```python
from build123d import *

# Parameters (mm, degrees)
SKETCH002_R  = 2.25
POCKET_DEPTH = 31.001
CHAMFER_SIZE = 2.5


with BuildPart() as chamfer_body:
    # Sketch → Loft section 0
    with BuildSketch(Plane.XY):
        with BuildLine():
            Line((-17, 0), (-38, 0))
            Line((-38, 0), (-38, -6))
            Line((-38, -6), (-20, -6))
            ThreePointArc((-16.27755, -9.477078), (-17.453105, -7.004482), (-20, -6))
            Line((-16.27755, -9.477078), (-15, -28.197751))
            ThreePointArc((-15, -28.197751), (-14.052596, -30.190467), (-12, -31))
            Line((-12, -31), (0, -31))
            Line((0, -31), (0, -27))
            ThreePointArc((-9.789322, -18.64486), (-6.435045, -24.627224), (0, -27))
            Line((-11.683183, -4.645958), (-9.789322, -18.64486))
            ThreePointArc((-11.683183, -4.645958), (-13.469651, -1.325133), (-17, 0))
        make_face()
    # Sketch001 → Loft section 1
    with BuildSketch(Plane.XY.offset(20)):
        with BuildLine():
            Line((-17, 0), (-38, 0))
            Line((-38, 0), (-38, -6))
            Line((-38, -6), (-16.5, -6))
            ThreePointArc((-12.77755, -9.220661), (-14.038837, -6.91692), (-16.5, -6))
            Line((-12.77755, -9.220661), (-11.623745, -17.1614))
            ThreePointArc((-11.623745, -17.1614), (-9.823458, -22.15833), (-6, -25.844998))
            ThreePointArc((-6, -25.844998), (-3.112034, -27.078665), (0, -27.5))
            Line((0, -27.5), (0, -24.5))
            ThreePointArc((-8.696641, -16.14486), (-6.029924, -22.072766), (0, -24.5))
            Line((-10.286118, -5.764115), (-8.696641, -16.14486))
            ThreePointArc((-10.286118, -5.764115), (-12.575601, -1.638712), (-17, 0))
        make_face()
    loft()

    # Sketch002 → Pocket (cut, through all)
    with BuildSketch(Plane(origin=(0, 0, 0), x_dir=(-1, 0, 0), z_dir=(0, 1, 0))):
        with Locations((23, 13.5)):
            Circle(SKETCH002_R)
        with Locations((31, 6.5)):
            Circle(SKETCH002_R)
    extrude(amount=-POCKET_DEPTH, mode=Mode.SUBTRACT)

    # Chamfer
    chamfer_edges = [chamfer_body.edges().sort_by_distance(p)[0] for p in [
        (-21.369261, -6, 15.050223),
        (-24.630739, -6, 11.949777),
        (-28.776606, -6, 6.844988),
        (-33.223394, -6, 6.155012),
    ]]
    chamfer(chamfer_edges, length=CHAMFER_SIZE)


with BuildPart() as part_mirroring:
    # Part__Mirroring: instance of Chamfer body
    add(chamfer_body.part.mirror(Plane(origin=(0, 0, 0), x_dir=(0, -1, 0), z_dir=(1, 0, 0))))


with BuildPart() as fusion:
    # Fusion base: copy of Chamfer body
    add(chamfer_body.part)

    # Fusion: union Part__Mirroring
    add(part_mirroring.part)


solid = fusion.part
```
Here's how the part is built. I have some questions about the finished solid (model axes, mm). Coordinates: 2 decimals unless noted, no trailing zeros. Return JSON: item names as keys, results as strings.
1) If we section it at A-A, the plane z = 12.25: Count the separate pieces of the cut face and the enclosed holes in it, then the cut area to 3 significant figures.
Results below:
{"separate pieces": "3", "enclosed holes": "0", "area": "500 mm²"}
2) Thinking about a two-plate mould opening in Z: for faces 1 (the face through (-27, 0, 10)), 2 (the face through (-25.146, -1.726, 14.176)), 3 (the face through (11, -9, 20)), which applies, +Z half, -Z half, draft (parallel to the pull), parting line (faces both ways), or undercut?
Results below:
{"face 1": "draft", "face 2": "undercut", "face 3": "+Z half"}
3) Will these pins go through, and if not, where does the flat tip stop? pin 1 (3 mm diameter, centred on y = -25, z = 11, fed in from -X); pin 2 (4 mm diameter, centred on y = -20.5, z = 5, fed in from -X) (3 decimals); pin 3 (10 mm diameter, centred on x = 9.5, z = 12.5, fed in from -Y); pin 4 (2.5 mm diameter, centred on x = 31, z = 6.5, fed in from +Y).
Results below:
{"pin 1": "x = -13.08", "pin 2": "x = -14.965", "pin 3": "y = -29.22", "pin 4": "through"}
4) I need wall thicknesses on line 1 (Z direction, x = 31, y = -2.6); line 2 (Z direction, x = 23, y = -2); line 3 (X direction, y = -1.75, z = 13.5). Which ranges of each line are inside material? Lowest first, please. Write a range as from..to.
Results below:
{"line 1": "0..4.25, 8.75..20", "line 2": "0..11.25, 15.75..20", "line 3": "-38..-25.25, -20.75..-12.63, 12.63..20.75, 25.25..38"}
